Model file for the job. Use its own axes, mm. Coordinates: 2 decimals unless noted, no trailing zeros. Write each loop counter-clockwise with the first axis right and the second up, starting at its lowest first coordinate (ties: lowest second). Pieces come first, ordered by that corner, then holes. Notation, with made-up numbers: M 67,15 L 92,15 A6 ccw 92,19 Z; hole C -32,-4.75 d7. An arc over 180 degrees is marked long. Put each result on its own line as item: value. Start each with the question number.
Q1. Drill centre lines: line 1 along X through (y, z) = (-23.5, -5); line 2 along X through (y, z) = (-9.5, -22.5); line 3 along Z through (x, y) = (-24, -0.75). Where is each one in solid material? Low to high.
Q2. Cut at A-A (x = 0). Write the cut outline in (y, z), then the cut area to 3 significant figures.
Q3. Drop flat-ended pins along their axis: pin 1 (1 mm diameter, centred on x = 2.5, z = 1.5, fed in from +Y); pin 2 (2 mm diameter, centred on x = -8, y = -21, fed in from +Z); pin 3 (4 mm diameter, centred on y = -21.5, z = 6, fed in from +X); pin 4 (3 mm diameter, centred on x = -7, y = -12.5, fed in from -Z). Give the stop position or say it passes through.
Q4. Cut at B-B (x = -24). Write the cut outline in (y, z).
Q5. Cut at C-C (x = -10). Write the cut outline in (y, z), then the cut area to 3 significant figures.
Q6. Pull direction X, two halves, no side cores. Call faces 1 (the cylindrical face through (-24.769, -12.878, 9.764)), 2 (the cylindrical face through (-24.12, -12.52, -18.49)), 3 (the flat face through (0, -25.4, 7)): pulls with the +X half, pulls with the -X half, needs draft (parallel to the pull), parting line crosses it, or undercut.
Q7. Cut at D-D (y = -10.5). Give the number of separate pieces and of enclosed holes in the cut face, then the cut area to 3 significant figures.
```python
from build123d import *

# Parameters (mm, degrees)
F0_R     = 30.3902596551
F1_DEPTH = 25.4
F2_R     = 2.6289
F3_DEPTH = 35.306
F4_R     = 1.651
F5_DEPTH = 25.4


# Not quite as in the source:
# - a feature names something its author has since deleted; it is built from what else it names


with BuildPart() as f1:
    # F0 (on Front) → F1 (new body)
    with BuildSketch(Plane.XZ):
        Circle(F0_R)
    extrude(amount=F1_DEPTH)

    # F2 (on face) → F3 (cut)
    with BuildSketch(Plane.XZ.offset(25.4)):
        with Locations((-9.1471226763, 23.6621449357)):
            Circle(F2_R)
        with Locations((0, 25.3564708744)):
            Circle(F2_R)
        with Locations((-20.2673863665, -15.1786801491)):
            Circle(F2_R)
        with Locations((-24.4002614445, -6.8444173004)):
            Circle(F2_R)
        with Locations((-25.2433696844, 2.4200180379)):
            Circle(F2_R)
        with Locations((-22.6828446466, 11.3634125374)):
            Circle(F2_R)
        with Locations((-17.0644994257, 18.7779112138)):
            Circle(F2_R)
        with Locations((-4.7339240202, -24.8319767568)):
            Circle(F2_R)
        with Locations((-13.4029121308, -21.4571821289)):
            Circle(F2_R)
        with Locations((4.5687830844, -24.847279318)):
            Circle(F2_R)
        with Locations((9.1414989998, 23.6320609235)):
            Circle(F2_R)
        with Locations((17.0427642284, 18.721806202)):
            Circle(F2_R)
        with Locations((22.6366860342, 11.2888638188)):
            Circle(F2_R)
        with Locations((25.1677742804, 2.33709383)):
            Circle(F2_R)
        with Locations((24.294191474, -6.9245176239)):
            Circle(F2_R)
        with Locations((20.1339198139, -15.2451385957)):
            Circle(F2_R)
        with Locations((13.2488270404, -21.5010231169)):
            Circle(F2_R)
    extrude(amount=-F3_DEPTH, mode=Mode.SUBTRACT)

    # F4 (on face) → F5 (cut)
    with BuildSketch(Plane.XZ.offset(25.4)):
        Circle(F4_R)
    extrude(amount=-F5_DEPTH, mode=Mode.SUBTRACT)


solid = f1.part
```
Computed values:
1. line 1: -29.98 to -26.27, -22.53 to 22.5, 26.09 to 29.98
1. line 2: -20.43 to -15.82, -10.99 to -5.95, -3.52 to 3.38, 5.75 to 10.82, 15.68 to 20.43
1. line 3: -18.64 to -9.44, -4.25 to 0.1, 4.74 to 9.09, 13.64 to 18.64
2. outline: M -25.4,-30.39 L 0,-30.39 L 0,-1.65 L -25.4,-1.65 Z; M -25.4,1.65 L 0,1.65 L 0,22.73 L -25.4,22.73 Z; M -25.4,27.99 L 0,27.99 L 0,30.39 L -25.4,30.39 Z
2. area: 1,330 mm2
3. pin 1: y = 0
3. pin 2: z = 29.57
3. pin 3: x = 30.13
3. pin 4: z = -29.89
4. outline: M -25.4,-18.64 L 0,-18.64 L 0,-9.44 L -25.4,-9.44 Z; M -25.4,-4.25 L 0,-4.25 L 0,0.1 L -25.4,0.1 Z; M -25.4,4.74 L 0,4.74 L 0,9.09 L -25.4,9.09 Z; M -25.4,13.64 L 0,13.64 L 0,18.64 L -25.4,18.64 Z
5. outline: M -25.4,-28.7 L 0,-28.7 L 0,21.18 L -25.4,21.18 Z; M -25.4,26.15 L 0,26.15 L 0,28.7 L -25.4,28.7 Z
5. area: 1,330 mm2
6. face 1: undercut
6. face 2: parting line crosses it
6. face 3: needs draft
7. separate pieces: 1
7. enclosed holes: 18
7. area: 2,520 mm2
